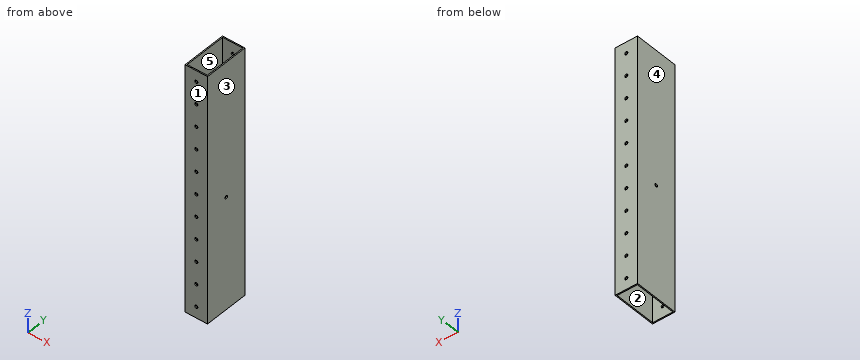
Autodesk Inventor part; units mm, degrees
ref_plane "YZ Plane" through (0, 0, 0) normal (1, 0, 0) x (0, 1, 0)
ref_plane "XZ Plane" through (0, 0, 0) normal (0, 1, 0) x (-1, 0, 0)
ref_plane "XY Plane" through (0, 0, 0) normal (0, 0, 1) x (1, 0, 0)
sketch "Sketch1" plane through (0, 0, 0) normal (0, 0, 1) x (1, 0, 0)
  line L0 (-12.1708, 16.0073) -> (13.2292, 16.0073)
  line L1 (13.2292, 16.0073) -> (13.2292, -34.7927)
  line L2 (13.2292, -34.7927) -> (-12.1708, -34.7927)
  line L3 (-12.1708, -34.7927) -> (-12.1708, 16.0073)
  line L4 (11.9592, 14.7373) -> (-10.9008, 14.7373)
  line L5 (-10.9008, 14.7373) -> (-10.9008, -33.5227)
  line L6 (-10.9008, -33.5227) -> (11.9592, -33.5227)
  line L7 (11.9592, -33.5227) -> (11.9592, 14.7373)
  point P0 (0, 0)
  dimension "d0" = 25.4
  dimension "d1" = 50.8
  dimension "d2" = 1.27
extrude "Extrusion1" add sketch "Sketch1" along normal blind 279.4
sketch "Sketch2" plane through (-12.1708, 16.0073, 0) normal (0, 1, 0) x (1, 0, 0)
  circle A0 centre (12.7, -12.7) radius 1.7272
  line L0 (25.4, 0) -> (0, 0)
  line L1 (0, 0) -> (0, -279.4)
  point P0 (12.1708, 0)
  dimension "d5" = 3.4544
  dimension "d6" = 12.7
  dimension "d7" = 12.7
extrude "Extrusion2" cut sketch "Sketch2" against normal through all
pattern_linear "Rectangular Pattern1" count 11 spacing 25.4 along (0, 0, 1) of "Extrusion2"
sketch "Sketch4" plane through (13.2292, -34.7927, 0) normal (1, 0, 0) x (0, 0, -1)
  circle A0 centre (-127, 25.4) radius 1.7272
  line L0 (-279.4, 0) -> (-279.4, 50.8)
  line L1 (0, 50.8) -> (-279.4, 50.8)
  point P0 (0, 34.7927)
  dimension "d21" = 3.4544
  dimension "d22" = 152.4
  dimension "d23" = 25.4
extrude "Extrusion4" cut sketch "Sketch4" against normal blind 25.4
equation "\"d3\" = d13"
equation "\"d13\" = 279.4"
properties part number "VerseFrame 11in w hole"
Source: CAD feature listing. Evaluate the final solid. Frame: model axes, mm. Face numbers are marked on the shaded views. A direction names the side the tool comes from. Coordinates: 2 decimals unless noted, no trailing zeros. Write each loop counter-clockwise with the first axis right and the second up, starting at its lowest first coordinate (ties: lowest second). Pieces come first, ordered by that corner, then holes. Notation, with made-up numbers: M 12.25,29.25 L 41.25,29.25 A31 cw 41.25,68.25 Z; hole C 1.5,78.25 d7. An arc over 180 degrees is marked long. Answer as a JSON object with one key per item and string values.
1. Draft query along Y for the marked faces 1, 2 and 3. Return one class per face: released by +Y, released by -Y, zero draft, split by the parting line, or undercut.
Evaluation:
{"face 1": "released by -Y", "face 2": "undercut", "face 3": "zero draft"}
2. Contact query for a flat-ended pin moving along its axis: P1, Ø3, axis at x = 0.53, z = 241.3, coming from the -Y side. Output: stop coordinate, or through.
Evaluation:
{"P1": "through"}
3. Cut plane A-A on y = 8. Output: boundary loops of the cut face in (x, z), plus the area to 3 significant figures.
Evaluation:
{"outline": "M -12.17,0 L -10.9,0 L -10.9,279.4 L -12.17,279.4 Z; M 11.96,0 L 13.23,0 L 13.23,279.4 L 11.96,279.4 Z", "area": "710 mm^2"}
4. Access query for the marked faces 4 and 5. Directions: +Z, -Z, +X, -X, +Y, -Y. A direction counts if a zero-diameter tool reaches every point of the face in a straight line with its end or side. Return the directions, or none.
Evaluation:
{"face 4": "+Z, -Z, -X, +Y, -Y", "face 5": "+Z, -Z"}
5. Ray query, L1, parallel to X at y = -34.5, z = 114.3; L2, parallel to X at y = -11.5, z = 32; L3, parallel to Y at x = 7, z = 61. Return the intervals inside material, ascending.
Evaluation:
{"L1": "-12.17 to -1.2, 2.26 to 13.23", "L2": "-12.17 to -10.9, 11.96 to 13.23", "L3": "-34.79 to -33.52, 14.74 to 16.01"}
6. Cut plane B-B on z = 183. Output: boundary loops of the cut face in (x, y), plus the area to 3 significant figures.
Evaluation:
{"outline": "M -12.17,-34.79 L 13.23,-34.79 L 13.23,16.01 L -12.17,16.01 Z; hole M -10.9,-33.52 L 11.96,-33.52 L 11.96,14.74 L -10.9,14.74 Z", "area": "187 mm^2"}
